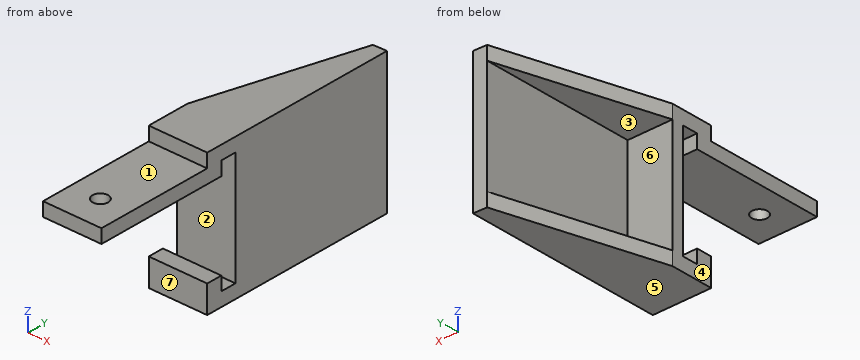
```python
from build123d import *

# Parameters (mm, degrees)
F0_W      = 30
F0_H      = 22
F1_DEPTH  = 72
F3_DEPTH  = 72.001
F4_DEPTH  = 7
F6_DEPTH  = 7
F7_W      = 8
F7_H      = 44
F8_DEPTH  = 30.001
F9_W      = 30
F9_H      = 7
F10_DEPTH = 60
F11_R     = 4
F12_DEPTH = 65.001


with BuildPart() as f1:
    # F0 (on Top) → F1 (new body)
    with BuildSketch(Plane.XY):
        with Locations((-15, 11)):
            Rectangle(F0_W, F0_H)
        Polygon((-6.99437, 101.719299), (-30, 22), (0, 22), (0, 102), align=None)
    extrude(amount=F1_DEPTH)

    # F2 (on face) → F3 (cut, through all)
    with BuildSketch(Plane.XY.offset(72)):
        Polygon((-6.99437, 101.719299), (-30, 22), (-7, 22), align=None)
    extrude(amount=-F3_DEPTH, mode=Mode.SUBTRACT)

    # F2 (on face) → F4 (join)
    with BuildSketch(Plane.XY.offset(72)):
        Polygon((-6.99437, 101.719299), (-30, 22), (-7, 22), align=None)
    extrude(amount=-F4_DEPTH)

    # F5 (on face) → F6 (join)
    with BuildSketch(Plane(origin=(0, 0, 0), x_dir=(1, 0, 0), z_dir=(0, 0, -1))):
        Polygon((-6.99437, -101.719299), (-7, -22), (-30, -22), align=None)
    extrude(amount=-F6_DEPTH)

    # F7 (on face) → F8 (cut, through all)
    with BuildSketch(Plane(origin=(-30, 0, 0), x_dir=(0, -1, 0), z_dir=(-1, 0, 0))):
        Polygon((-8, 65), (-16, 65), (-16, 7), (-8, 7), (-8, 14), (-8, 58), align=None)
        with Locations((-4, 36)):
            Rectangle(F7_W, F7_H)
    extrude(amount=-F8_DEPTH, mode=Mode.SUBTRACT)

    # F9 (on face) → F10 (join)
    with BuildSketch(Plane.XZ):
        with Locations((-15, 61.5)):
            Rectangle(F9_W, F9_H)
    extrude(amount=F10_DEPTH)

    # F11 (on face) → F12 (cut, through all)
    with BuildSketch(Plane.XY.offset(65)):
        with Locations((-15, -44)):
            Circle(F11_R)
    extrude(amount=-F12_DEPTH, mode=Mode.SUBTRACT)


solid = f1.part
```
Read the model definition and answer for the solid it produces. Units are mm, in the model's axes. Face numbers are marked on the shaded views. A direction names the side the tool comes from. Give positions to 0.01 mm unless a question says otherwise; leave off trailing zeros. Order: outer loops, then holes, each group sorted by start corner. A loop starts at its lowest first (then second) coordinate and runs counter-clockwise, first axis right, second up. Notation, with made-up numbers: (-7.5, 22) -> (19.5, 22) arc R30 ccw to (19.5, 60) -> close; hole circle Ø5 at (-37.5, 20.5). An arc over 180 degrees is marked (long way). One line per item, written item: value. Start each with the question number.
(1) The part is cut by section A-A (x = -15.5). Determine the outline of the cut face in (y, z).
(2) For a pull along Z with two mould halves and no side action, classify the marked faces 1, 2, 3 and 4 as released by +Z, released by -Z, zero draft, split by the parting line, or undercut.
(3) The part is cut by section B-B (y = -44). Determine the outline of the cut face in (x, z).
(4) The part is cut by section D-D (y = 85.5). Determine the outline of the cut face in (x, z).
(5) Flat-ended cylindrical pins translate along their axes: P1, Ø3, axis at x = -10, z = 18.5, coming from the +Y side; P2, Ø3.5, axis at x = -12.5, z = 69.5, coming from the -Y side; P3, Ø9, axis at x = -22, y = -22, coming from the +Z side; P4, Ø12, axis at y = -9.5, z = 13.5, coming from the -X side (1 decimal). Find the tip coordinate at first contact, or state that the pin passes through.
(6) Straight lines are drawn through the part: L1, parallel to Y at x = -15, z = 62; L2, parallel to Z at x = -6, y = 10.5; L3, parallel to Y at x = -26, z = 12. For each, find the intervals that lie inside material, in ascending order.
(7) The part is cut by section C-C (z = 22). Determine the outline of the cut face in (x, y).
(8) A tool of negligible diameter and unlimited length cuts with its end or side. For the marked faces 5, 6 and 7, from which of +Z, -Z, +X, -X, +Y, -Y can it reach the whole face along a straight path? Write none if from no direction.
Taken from the geometry:
1. outline: (-60, 58) -> (-47.97, 58) -> (-47.97, 65) -> (-60, 65) -> close; (-40.03, 58) -> (8, 58) -> (8, 65) -> (16, 65) -> (16, 7) -> (8, 7) -> (8, 14) -> (0, 14) -> (0, 0) -> (72.25, 0) -> (72.25, 7) -> (22, 7) -> (22, 65) -> (72.25, 65) -> (72.25, 72) -> (0, 72) -> (0, 65) -> (-40.03, 65) -> close
2. face 1: released by +Z
2. face 2: undercut
2. face 3: undercut
2. face 4: zero draft
3. outline: (-30, 58) -> (-19, 58) -> (-19, 65) -> (-30, 65) -> close; (-11, 58) -> (0, 58) -> (0, 65) -> (-11, 65) -> close
4. outline: (-11.67, 0) -> (0, 0) -> (0, 72) -> (-11.67, 72) -> (-11.67, 65) -> (-7, 65) -> (-7, 7) -> (-11.67, 7) -> close
5. P1: y = 22
5. P2: y = 0
5. P3: z = 65
5. P4: through
6. L1: -60 to -48, -40 to 8, 16 to 22
6. L2: 0 to 7, 65 to 72
6. L3: 0 to 8, 16 to 22
7. outline: (-30, 16) -> (0, 16) -> (0, 102) -> (-6.99, 101.72) -> (-7, 22) -> (-30, 22) -> close
8. face 5: -Z, +X, -X, +Y, -Y
8. face 6: -X, +Y
8. face 7: -Z, +X, -X, -Y
